Design review of the part built by this model. Coordinates are the model's own, in mm. A direction names the side the tool comes from. Round coordinates to 2 decimals unless told otherwise and drop trailing zeros. Write each loop counter-clockwise with the first axis right and the second up, starting at its lowest first coordinate (ties: lowest second). Pieces come first, ordered by that corner, then holes. Notation, with made-up numbers: (82, -7) -> (125, -7) arc R12 ccw to (125, 6) -> close; hole circle Ø10 at (51, 88). An arc over 180 degrees is marked (long way). Write item = value, one per line. Start each with the question number.
Item 1: Add section B-B, the plane z = -12.7. State the section outline as (x, y) points, then the cut area to 3 significant figures.
Item 2: For pin 1 Ø1.5 at (x, z) = (2, -66.5) entering from +Y; pin 2 Ø3 at (y, z) = (6.35, -12.7) entering from -X; pin 3 Ø0.9 at (x, z) = (2, -61.5) entering from -Y; pin 4 Ø1.5 at (x, y) = (2.5, 7.5) entering from -Z, all flat-tipped, find the tip position at first contact; note any pin that passes through.
Item 3: Add section D-D, the plane x = 1.7. State the section outline as (y, z) points (3 decimals).
Item 4: Add section C-C, the plane y = 6.35. State the section outline as (x, z) points.
Item 5: Add section A-A, the plane z = -31.75. State the section outline as (x, y) points.
Item 6: Machinability: for faces 4 (the flat face through (1, -2, -116.408)), 5 (the flat face through (1, 16, -25.4)), 6 (the flat face through (1, 31.75, -59)), which of the approach directions +Z, -Z, +X, -X, +Y, -Y give a long, thin tool a straight path to every point of the face, cutting with its end or side? Answer none if there is none.
Item 7: Mouldability with a two-part tool opening along Z and no side actions: class faces 1 (the flat face through (1, 6, 0)), 2 (the cylindrical face through (1.532, 5.372, -15.058)), 3 (the flat face through (1, 19.05, -13)) as released by +Z, released by -Z, zero draft, split by the parting line, or undercut.
Item 8: To check wall thickness, follow L1, parallel to Y at x = 1.2, z = -12.7; L2, parallel to Z at x = 1, y = 24.5; L3, parallel to Z at x = 1.35, y = 24. State the ranges of each line that lie inside material, in increasing order.
from build123d import *

# Parameters (mm, degrees)
SKETCH2_2_R         = 2.0193
BOSS_EXTRUDE2_DEPTH = 3.0226
SKETCH6_R           = 2.5527
CUT_EXTRUDE4_DEPTH  = 4.0226


with BuildPart() as part:
    # Sketch2<2> → Boss-Extrude2 (new body)
    with BuildSketch(Plane(origin=(0, 0, 0), x_dir=(0, 0, -1), z_dir=(1, 0, 0))):
        Polygon((0, 0), (0, 12.7), (25.4, 12.7), (25.4, 19.05), (0, 19.05), (0, 31.75), (38.1, 31.75), (116.4082, 31.75), (116.4082, 34.7472), (162.99536189, 34.7472), (176.7332, -2.9972), (116.4082, -2.9972), (116.4082, 0), (38.1, 0), align=None)
        with Locations((12.7, 25.4)):
            Circle(SKETCH2_2_R, mode=Mode.SUBTRACT)
        with Locations((12.7, 6.35)):
            Circle(SKETCH2_2_R, mode=Mode.SUBTRACT)
        with Locations((31.75, 15.875)):
            Circle(SKETCH2_2_R, mode=Mode.SUBTRACT)
    extrude(amount=BOSS_EXTRUDE2_DEPTH)

    # Sketch6 → Cut-Extrude4 (cut, through all)
    with BuildSketch(Plane(origin=(3.0226, 0, 0), x_dir=(0, 0, -1), z_dir=(1, 0, 0))):
        with Locations((12.7, 25.4)):
            Circle(SKETCH6_R)
        with Locations((31.75, 15.875)):
            Circle(SKETCH6_R)
        with Locations((12.7, 6.35)):
            Circle(SKETCH6_R)
    extrude(amount=-CUT_EXTRUDE4_DEPTH, mode=Mode.SUBTRACT)


solid = part.part
Result set:
q1.outline = (0, 0) -> (3.02, 0) -> (3.02, 3.8) -> (0, 3.8) -> close; (0, 8.9) -> (3.02, 8.9) -> (3.02, 12.7) -> (0, 12.7) -> close; (0, 19.05) -> (3.02, 19.05) -> (3.02, 22.85) -> (0, 22.85) -> close; (0, 27.95) -> (3.02, 27.95) -> (3.02, 31.75) -> (0, 31.75) -> close
q1.area = 45.9 mm²
q2.pin_1 = 31.75
q2.pin_2 = through
q2.pin_3 = 0
q2.pin_4 = -173.19
q3.outline = (-2.997, -176.733) -> (34.747, -162.995) -> (34.747, -116.408) -> (31.75, -116.408) -> (31.75, 0) -> (19.05, 0) -> (19.05, -25.4) -> (12.7, -25.4) -> (12.7, 0) -> (0, 0) -> (0, -116.408) -> (-2.997, -116.408) -> close; hole circle Ø5.105 at (6.35, -12.7); hole circle Ø5.105 at (15.875, -31.75); hole circle Ø5.105 at (25.4, -12.7)
q4.outline = (0, -173.33) -> (3.02, -173.33) -> (3.02, -15.25) -> (0, -15.25) -> close; (0, -10.15) -> (3.02, -10.15) -> (3.02, 0) -> (0, 0) -> close
q5.outline = (0, 0) -> (3.02, 0) -> (3.02, 13.32) -> (0, 13.32) -> close; (0, 18.43) -> (3.02, 18.43) -> (3.02, 31.75) -> (0, 31.75) -> close
q6.face_4 = +Z, +X, -X, -Y
q6.face_5 = +Z, +X, -X
q6.face_6 = +Z, +X, -X, +Y
q7.face_1 = released by +Z
q7.face_2 = undercut
q7.face_3 = zero draft
q8.L1 = 0 to 3.8, 8.9 to 12.7, 19.05 to 22.85, 27.95 to 31.75
q8.L2 = -166.73 to -15.09, -10.31 to 0
q8.L3 = -166.91 to -14.83, -10.57 to 0
